from build123d import *

# Parameters (mm, degrees)
F0_R           = 25
F0_R_2         = 6
F1_DEPTH       = 2
F2_DEPTH       = 7.5
F5_D           = 4
F5_CSINK_D     = 7
F5_CSINK_ANGLE = 90


# Not quite as in the source:
# - a feature names something its author has since deleted; it is built from what else it names


with BuildPart() as f1:
    # F0 (on Top) → F1 (new body)
    with BuildSketch(Plane.XY):
        Circle(F0_R)
        with BuildLine():
            ThreePointArc((0, 11), (7.7781745931, 7.7781745931), (11, 0))
            ThreePointArc((11, 0), (8.9302855497, -6.4226162893), (3.5, -10.4283268073))
            Line((3.5, -10.4283268073), (3.5, -13))
            Line((3.5, -13), (0, -13))
            Line((0, -13), (0, -11))
            ThreePointArc((0, -11), (-10.9277987049, -1.258258902), (-2.5, 10.7121426428))
            Line((-2.5, 10.7121426428), (-2.5, 13))
            Line((-2.5, 13), (0, 13))
            Line((0, 13), (0, 11))
        make_face(mode=Mode.SUBTRACT)
        with BuildLine():
            ThreePointArc((3.5, -10.4283268073), (8.9302855497, -6.4226162893), (11, 0))
            ThreePointArc((11, 0), (7.7781745931, 7.7781745931), (0, 11))
            ThreePointArc((0, 11), (-1.258258902, 10.9277987049), (-2.5, 10.7121426428))
            ThreePointArc((-2.5, 10.7121426428), (-10.9277987049, -1.258258902), (0, -11))
            ThreePointArc((0, -11), (1.773189939, -10.8561410013), (3.5, -10.4283268073))
        make_face()
        Circle(F0_R_2, mode=Mode.SUBTRACT)
        Circle(F0_R_2)
        with BuildLine():
            ThreePointArc((-2.5, 10.7121426428), (-1.258258902, 10.9277987049), (0, 11))
            Line((0, 11), (0, 13))
            Line((0, 13), (-2.5, 13))
            Line((-2.5, 13), (-2.5, 10.7121426428))
        make_face()
        with BuildLine():
            Line((3.5, -13), (3.5, -10.4283268073))
            ThreePointArc((3.5, -10.4283268073), (1.773189939, -10.8561410013), (0, -11))
            Line((0, -11), (0, -13))
            Line((0, -13), (3.5, -13))
        make_face()
    extrude(amount=F1_DEPTH)

    # F0 (on Top) → F2 (join)
    with BuildSketch(Plane.XY):
        with BuildLine():
            ThreePointArc((3.5, -10.4283268073), (8.9302855497, -6.4226162893), (11, 0))
            ThreePointArc((11, 0), (7.7781745931, 7.7781745931), (0, 11))
            ThreePointArc((0, 11), (-1.258258902, 10.9277987049), (-2.5, 10.7121426428))
            ThreePointArc((-2.5, 10.7121426428), (-10.9277987049, -1.258258902), (0, -11))
            ThreePointArc((0, -11), (1.773189939, -10.8561410013), (3.5, -10.4283268073))
        make_face()
        Circle(F0_R_2, mode=Mode.SUBTRACT)
        with BuildLine():
            Line((3.5, -13), (3.5, -10.4283268073))
            ThreePointArc((3.5, -10.4283268073), (1.773189939, -10.8561410013), (0, -11))
            Line((0, -11), (0, -13))
            Line((0, -13), (3.5, -13))
        make_face()
        with BuildLine():
            ThreePointArc((-2.5, 10.7121426428), (-1.258258902, 10.9277987049), (0, 11))
            Line((0, 11), (0, 13))
            Line((0, 13), (-2.5, 13))
            Line((-2.5, 13), (-2.5, 10.7121426428))
        make_face()
    extrude(amount=F2_DEPTH)

    # F5 (through all)
    with Locations(Plane(origin=(0, 0, 0), x_dir=(1, 0, 0), z_dir=(0, 0, -1))):
        with Locations((-8.5, 0), (8.5, 0)):
            CounterSinkHole(F5_D / 2, F5_CSINK_D / 2, counter_sink_angle=F5_CSINK_ANGLE)


solid = f1.part
Verification items for the finished model (mm, model axes). A direction names the side the tool comes from. Round coordinates to 2 decimals unless told otherwise and drop trailing zeros. Order: outer loops, then holes, each group sorted by start corner. A loop starts at its lowest first (then second) coordinate and runs counter-clockwise, first axis right, second up. Notation, with made-up numbers: (-40, 72.25) -> (-36, 72.25) arc R23 cw to (-36, 87.25) -> close; hole circle Ø2 at (-15.5, -3.5). An arc over 180 degrees is marked (long way). Put each result on its own line as item: value.
1) Mould release check, pull along X, two halves, no side actions. Record for faces 1 (the conical face through (-10, -2, 1)), 2 (the cylindrical face through (-10.95, -1.04, 4.71)), 3 (the flat face through (5, -11, 2)): +X half, -X half, draft (parallel to the pull), parting line (faces both ways), or undercut.
Final values:
face 1: undercut
face 2: -X half
face 3: draft
2) Set-up check for faces 4 (the flat face through (0, -12, 5)), 5 (the flat face through (0, 12, 5)), 6 (the flat face through (0, 0, 2)): record each of +Z, -Z, +X, -X, +Y, -Y from which the full face is reachable in a straight line by a thin tool's end or side.
Final values:
face 4: +Z, -X, -Y
face 5: +Z, +X, +Y
face 6: +Z
3) Section check C-C (x = -8.5). Record the cut outline in (y, z).
Final values:
outline: (-23.51, 0) -> (-3.5, 0) -> (-2, 1.5) -> (-2, 7.5) -> (-6.98, 7.5) -> (-6.98, 2) -> (-23.51, 2) -> close; (2, 1.5) -> (3.5, 0) -> (23.51, 0) -> (23.51, 2) -> (6.98, 2) -> (6.98, 7.5) -> (2, 7.5) -> close
4) Section check D-D (x = 15). Record the cut outline in (y, z).
Final values:
outline: (-20, 0) -> (20, 0) -> (20, 2) -> (-20, 2) -> close
5) Section check B-B (z = 4.75). Record the cut outline in (x, y).
Final values:
outline: (-2.5, 10.71) arc R11 ccw to (0, -11) -> (0, -13) -> (3.5, -13) -> (3.5, -10.43) arc R11 ccw to (0, 11) -> (0, 13) -> (-2.5, 13) -> close; hole circle Ø4 at (-8.5, 0); hole circle Ø12 at (0, 0); hole circle Ø4 at (8.5, 0)
6) Depth check by flat-ended pin: pin 1 (1.3 mm diameter, centred on y = -12, z = 5.5, fed in from +X); pin 2 (0.8 mm diameter, centred on x = -1, z = 4.5, fed in from +Y); pin 3 (1 mm diameter, centred on x = -10.5, z = 3.5, fed in from +Y); pin 4 (3.5 mm diameter, centred on x = -8.5, y = 0, fed in from +Z). Enter the tip coordinate at first touch or a pass-through.
Final values:
pin 1: stops at x = 3.5
pin 2: stops at y = 13
pin 3: stops at y = 4.58
pin 4: passes through
7) Material ranges on line 1 (X direction, y = -0.5, z = 6.5); line 2 (Z direction, x = 3.5, y = 1); line 3 (X direction, y = -1, z = 3), recorded low to high.
Final values:
line 1: x = -10.99 to -10.44, -6.56 to -5.98, 5.98 to 6.56, 10.44 to 10.99
line 2: z = 0 to 2
line 3: x = -10.95 to -10.23, -6.77 to -5.92, 5.92 to 6.77, 10.23 to 10.95
8) Section check A-A (y = 0). Record the cut outline in (x, z), then the cut area to 3 significant figures.
Final values:
outline: (-25, 0) -> (-12, 0) -> (-10.5, 1.5) -> (-10.5, 7.5) -> (-11, 7.5) -> (-11, 2) -> (-25, 2) -> close; (-6.5, 1.5) -> (-5, 0) -> (5, 0) -> (6.5, 1.5) -> (6.5, 7.5) -> (6, 7.5) -> (6, 2) -> (-6, 2) -> (-6, 7.5) -> (-6.5, 7.5) -> close; (10.5, 1.5) -> (12, 0) -> (25, 0) -> (25, 2) -> (11, 2) -> (11, 7.5) -> (10.5, 7.5) -> close
area: 90.5 mm^2
